Read the model definition and answer for the solid it produces. Units are mm, in the model's axes. A direction names the side the tool comes from. Coordinates: 2 decimals unless noted, no trailing zeros. Write each loop counter-clockwise with the first axis right and the second up, starting at its lowest first coordinate (ties: lowest second). Pieces come first, ordered by that corner, then holes.
Autodesk Inventor part; units mm, degrees
ref_plane "YZ Plane" through (0, 0, 0) normal (1, 0, 0) x (0, 1, 0)
ref_plane "XZ Plane" through (0, 0, 0) normal (0, 1, 0) x (-1, 0, 0)
ref_plane "XY Plane" through (0, 0, 0) normal (0, 0, 1) x (1, 0, 0)
sketch "Sketch1" plane through (0, 0, 0) normal (0, 0, 1) x (1, 0, 0)
  line L0 (-19.15, 21.15) -> (19.15, 21.15)
  line L1 (21.15, 19.15) -> (21.15, -19.15)
  line L2 (19.15, -21.15) -> (-19.15, -21.15)
  line L3 (-21.15, -19.15) -> (-21.15, 19.15)
  line L4 (-19.15, 21.15) -> (-21.15, 19.15)
  line L5 (-19.15, -21.15) -> (-21.15, -19.15)
  line L6 (21.15, -19.15) -> (19.15, -21.15)
  line L7 (19.15, 21.15) -> (21.15, 19.15)
  point P0 (0, 0)
  point P1 (-21.15, 21.15)
  point P2 (21.15, -21.15)
  point P3 (21.15, 21.15)
  point P4 (-21.15, -21.15)
  point P5 (-21.15, 0)
  point P6 (0, 21.15)
  dimension "d0" = 2
  dimension "d1" = 2
  dimension "d2" = 2
  dimension "d3" = 2
  dimension "d4" = 2
  dimension "d5" = 2
  dimension "d6" = 2
  dimension "d7" = 2
  dimension "d8" = 42.3
  dimension "d9" = 42.3
extrude "Extrusion1" add sketch "Sketch1" along normal blind 44.2
sketch "Sketch2" plane through (0, 0, 44.2) normal (0, 0, 1) x (1, 0, 0)
  circle A0 centre (0, 0) radius 18
  dimension "d12" = 36
extrude "Extrusion2" add sketch "Sketch2" along normal blind 24.5
sketch "Sketch3" plane through (0, 0, 68.7) normal (0, 0, 1) x (1, 0, 0)
  circle A0 centre (0, 0) radius 11
  dimension "d15" = 22
extrude "Extrusion3" add sketch "Sketch3" along normal blind 2
sketch "Sketch4" plane through (0, 0, 70.7) normal (0, 0, 1) x (1, 0, 0)
  circle A0 centre (0, 0) radius 4
  line L0 (-2.6458, 3) -> (2.6458, 3)
  dimension "d18" = 8
  dimension "d19" = 7
extrude "Extrusion4" add sketch "Sketch4" along normal blind 17.5 contours A0 L0 picked at (-1.0918, 0.7386)
extrude "Extrusion5" add sketch "Sketch4" along normal blind 2.3 contours L0 A0 picked at (-0.6179, 3.1815)
equation "\"d9\" = d8"
properties part number "Gearmotor"
Item 1: The part is cut by section B-B (y = 0). Give the vertices of the cut face in (x, z).
Item 2: The part is cut by section C-C (z = 65.5). Give the vertices of the cut face in (x, y).
Item 3: The part is cut by section D-D (y = 12). Give the vertices of the cut face in (x, z), and give its area (3 significant figures).
Item 4: Given pin 1 (12 mm diameter, centred on y = 4.5, z = 67.5, fed in from -X); pin 2 (2 mm diameter, centred on x = -0.5, z = 67.5, fed in from -Y); pin 3 (0.5 mm diameter, centred on x = 1, y = 3.5, fed in from +Z), each flat-ended and moving along its own axis, determine where each tip first touches the part or whether it passes through.
Item 5: The part is cut by section A-A (x = 0). Give the vertices of the cut face in (y, z), and give its area (3 significant figures).
Item 6: Find the intervals of material crossed by probe 1 along Z at (x, y) = (-2, 15); probe 2 along Z at (x, y) = (9, -3.5); probe 3 along X at (y, z) = (12.5, 65), in increasing order.
Item 7: For faces 1 (the flat face through (0, 3, 80)), 2 (the flat face through (20.2, -20.1, 21.8)), 3 (the flat face through (0, -5, 70.7)), determine the directions among +Z, -Z, +X, -X, +Y, -Y from which every point of the face is accessible in a straight line to the end or side of a thin tool.
Answer:
1. outline: (-21.15, 0) - (21.15, 0) - (21.15, 44.2) - (18, 44.2) - (18, 68.7) - (11, 68.7) - (11, 70.7) - (4, 70.7) - (4, 88.2) - (-4, 88.2) - (-4, 70.7) - (-11, 70.7) - (-11, 68.7) - (-18, 68.7) - (-18, 44.2) - (-21.15, 44.2) - close
2. outline: circle Ø36 at (0, 0)
3. outline: (-21.15, 0) - (21.15, 0) - (21.15, 44.2) - (13.42, 44.2) - (13.42, 68.7) - (-13.42, 68.7) - (-13.42, 44.2) - (-21.15, 44.2) - close
3. area: 2,530 mm2
4. pin 1: stops at x = -18
4. pin 2: stops at y = -18
4. pin 3: stops at z = 73
5. outline: (-21.15, 0) - (21.15, 0) - (21.15, 44.2) - (18, 44.2) - (18, 68.7) - (11, 68.7) - (11, 70.7) - (4, 70.7) - (4, 73) - (3, 73) - (3, 88.2) - (-4, 88.2) - (-4, 70.7) - (-11, 70.7) - (-11, 68.7) - (-18, 68.7) - (-18, 44.2) - (-21.15, 44.2) - close
5. area: 2,920 mm2
6. probe 1: z = 0 to 68.7
6. probe 2: z = 0 to 70.7
6. probe 3: x = -12.95 to 12.95
7. face 1: +Z, +X, -X, +Y
7. face 2: +Z, -Z, +X, -Y
7. face 3: +Z
